Input: part model. Units: mm. Frame: model coordinates. A direction names the side the tool comes from. Round coordinates to 2 decimals unless told otherwise and drop trailing zeros. Use one line per item in the form item = value. Start each with the question number.
```python
from build123d import *

# Parameters (mm, degrees)
BOSS_EXTRUDE1_DEPTH      = 15
BOSS_EXTRUDE1_DEPTH_BACK = 15
BOSS_EXTRUDE2_DEPTH      = 30
CIRPATTERN1_COUNT        = 19
CIRPATTERN1_ANGLE        = 342


with BuildPart() as part:
    # Sketch2 → Boss-Extrude1 (new, two sides: drawn at the far end of the back side and taken through both)
    with BuildSketch(Plane.XY.offset(-BOSS_EXTRUDE1_DEPTH_BACK)):
        with BuildLine():
            ThreePointArc((0, 32.558207974), (-217.441792026, 250), (0, 467.441792026))
            Line((0, 467.441792026), (0, 500))
            ThreePointArc((0, 500), (-250, 250), (0, 0))
            Line((0, 0), (0, 32.558207974))
        make_face()
        with BuildLine():
            Line((0, 500), (0, 467.441792026))
            ThreePointArc((0, 467.441792026), (153.754565655, 403.754565655), (217.441792026, 250))
            ThreePointArc((217.441792026, 250), (153.754565655, 96.245434345), (0, 32.558207974))
            Line((0, 32.558207974), (0, 0))
            ThreePointArc((0, 0), (176.776695297, 73.223304703), (250, 250))
            ThreePointArc((250, 250), (176.776695297, 426.776695297), (0, 500))
        make_face()
        with BuildLine():
            Line((0, 312.5), (0, 260))
            Line((0, 260), (0, 240))
            Line((0, 240), (0, 187.5))
            ThreePointArc((0, 187.5), (44.194173824, 205.805826176), (62.5, 250))
            ThreePointArc((62.5, 250), (44.194173824, 294.194173824), (0, 312.5))
        make_face()
        with BuildLine():
            Line((0, 240), (0, 260))
            Line((0, 260), (0, 312.5))
            ThreePointArc((0, 312.5), (-62.5, 250), (0, 187.5))
            Line((0, 187.5), (0, 240))
        make_face()
    extrude(amount=BOSS_EXTRUDE1_DEPTH + BOSS_EXTRUDE1_DEPTH_BACK)

    # Sketch4 → Boss-Extrude2 (add)
    with BuildSketch(Plane.XY.offset(15)):
        with BuildLine():
            ThreePointArc((-62.043119193, 242.456700933), (-62.499642772, 249.788686637), (-62.092708437, 257.123591721))
            Line((-62.092708437, 257.123591721), (-217.325073014, 257.123591721))
            add(Edge.make_bspline(
                [(-217.325073014, 257.123591721), (-218.805807348, 249.792999154), (-217.310909893, 242.456700933)],
                knots=[0, 0, 0, 1, 1, 1], degree=2))
            Line((-217.310909893, 242.456700933), (-62.043119193, 242.456700933))
        make_face()
    boss_extrude2 = extrude(amount=-BOSS_EXTRUDE2_DEPTH)

    # CirPattern1: Boss-Extrude2 ×19 about axis
    cirpattern1_axis = Axis((0, 250, 0), (0, 0, 1))
    for i in range(1, CIRPATTERN1_COUNT):
        add(boss_extrude2.rotate(cirpattern1_axis, i * CIRPATTERN1_ANGLE / (CIRPATTERN1_COUNT - 1)))

    # Sketch1 → Cut-Revolve1 (revolve, cut)
    with BuildSketch(Plane(origin=(0, 0, 0), x_dir=(0, 0, -1), z_dir=(1, 0, 0)), mode=Mode.PRIVATE) as cut_revolve1_sk:
        with BuildLine():
            Line((-10, 0), (-10, -1.402735917))
            Line((-10, -1.402735917), (10, -1.402735917))
            Line((10, -1.402735917), (10, 0))
            add(Edge.make_bspline(
                [(10, 0), (10, 3), (0, 3), (-10, 3), (-10, 0)],
                knots=[0, 0, 0, 1.570796327, 1.570796327, 3.141592654, 3.141592654, 3.141592654], degree=2, weights=[1, 0.707106781, 1, 0.707106781, 1]))
        make_face()
    revolve(cut_revolve1_sk.sketch.rotate(Axis((0, 250, 0), (0, 0, 1)), 270), axis=Axis((0, 250, 0), (0, 0, 1)), mode=Mode.SUBTRACT)


solid = part.part
```
Item 1: First-contact query: pin 1 (8 mm diameter, centred on y = 78, z = -1.5, fed in from +X); pin 2 (15 mm diameter, centred on x = -141.5, z = -7.5, fed in from +Y); pin 3 (3 mm diameter, centred on x = -148, z = 10, fed in from +Y). Flat tips, straight axial feed; report the tip coordinate or a pass-through.
Item 2: Draft query along Y for faces 1 (the face through (-2, 254, 15)), 2 (the face through (-193.155, 349.86, -0.21)). Return one class per face: +Y half, -Y half, draft (parallel to the pull), parting line (faces both ways), or undercut.
Item 3: Ray query, line 1 (X direction, y = 68.5, z = -6.5); line 2 (Y direction, x = 168, z = 5.75); line 3 (X direction, y = 72.5, z = 7.25). Return the intervals inside material, ascending. Write a range as from..to.
Item 4: Reachability of faces 3 (the face through (-86.14, 50.35, -0.21)), 4 (the face through (-2, 254, -15)) from +Z, -Z, +X, -X, +Y, -Y: full face, straight path, thin tool, end or side. Return the list, or none.
Item 5: Cut plane A-A (x = 111). Give the number of separate pieces and of enclosed holes in the cut face, plus the area to 3 significant figures.
Final values:
q1.pin_1 = 181.12
q1.pin_2 = 460.78
q1.pin_3 = 452.58
q2.face_1 = draft
q2.face_2 = undercut
q3.line_1 = -168.59..-108.87, -52.59..-37.48, 8.73..23.45, 73.01..89.07, 119.74..168.59
q3.line_2 = 68.19..111.95, 152.6..169.22, 216.18..231.03, 272.39..287.28, 334.98..351.75, 388.05..431.81
q3.line_3 = -173.1..-125.6, -123.76..-106.28, -51.6..-36.48, 8.38..23.1, 71.23..87.29, 125.6..173.1
q4.face_3 = +Z, -Z
q4.face_4 = -Z, +X, -X, +Y, -Y
q5.separate_pieces = 8
q5.enclosed_holes = 0
q5.area = 5,310 mm^2
